Autodesk Inventor part; units mm, degrees
ref_plane "YZ Plane" through (0, 0, 0) normal (1, 0, 0) x (0, 1, 0)
ref_plane "XZ Plane" through (0, 0, 0) normal (0, 1, 0) x (-1, 0, 0)
ref_plane "XY Plane" through (0, 0, 0) normal (0, 0, 1) x (1, 0, 0)
sketch "Sketch1" plane through (0, 0, 0) normal (0, 1, 0) x (-1, 0, 0)
  circle A0 centre (0, 0) radius 10
  dimension "d0" = 20
extrude "Extrusion1" add sketch "Sketch1" along normal blind 15
sketch "Sketch2" plane through (0, 0, 0) normal (0, -1, 0) x (1, 0, 0)
  circle A0 centre (0, 0) radius 7.5
  dimension "d3" = 15
extrude "Extrusion2" cut sketch "Sketch2" against normal blind 5
fillet "Fillet1" radius 2 1 edges at (10, 15, 0)
sketch "Sketch3" plane through (0, 15, 0) normal (0, 1, 0) x (1, 0, 0)
  line L0 (-0.048, -4.9874) -> (-1.048, -4.9874)
  line L1 (-1.048, -4.9874) -> (-1.048, 2.5126)
  line L2 (-1.048, 2.5126) -> (-2.048, 2.5126)
  line L3 (-2.048, 2.5126) -> (-0.048, 5.0126)
  line L4 (-0.048, 5.0126) -> (-0.048, -4.9874)
  line L5 (-0.048, -4.9874) -> (0.952, -4.9874)
  line L6 (0.952, -4.9874) -> (0.952, 2.5126)
  line L7 (0.952, 2.5126) -> (1.952, 2.5126)
  line L8 (1.952, 2.5126) -> (-0.048, 5.0126)
  point P0 (0, 0)
  dimension "d7" = 1
  dimension "d8" = 7.5
  dimension "d9" = 10
extrude "Extrusion3" add sketch "Sketch3" along normal blind 0.5
properties part number "Device Direction Button"
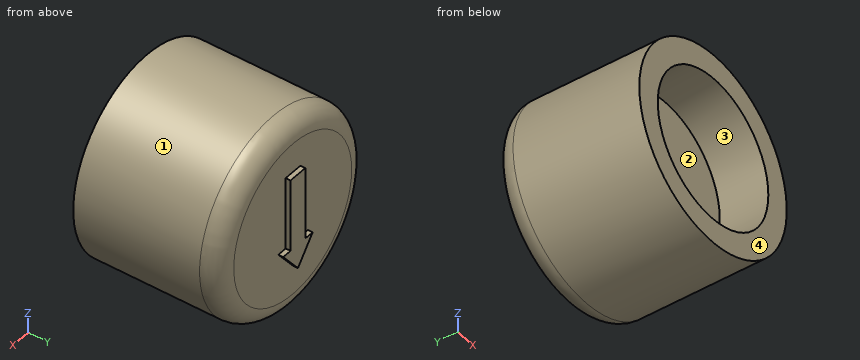
Input: part model. Units: mm. Frame: model coordinates. Face numbers are marked on the shaded views. Round coordinates to 2 decimals unless told otherwise and drop trailing zeros. Loops run counter-clockwise (first coordinate to the right, second up) from the corner with the lowest first, then second, coordinate; pieces in that order, holes last. Notation, with made-up numbers: M 18,31 L 22,31 A24 ccw 22,48 Z; hole C 69.5,-7 d3. An arc over 180 degrees is marked long. Answer in a Markdown table with one row per item. Add a question column.
1. Section A-A (z = 0). Output: boundary loops of the cut face in (x, y), and give its area (3 significant figures).
2. Section C-C (y = 11). Output: boundary loops of the cut face in (x, z), and give its area (3 significant figures).
3. Section B-B (y = 1). Output: boundary loops of the cut face in (x, z).
4. Mould query, pull axis Z, two halves, no side actions, for the marked faces 1, 2, 3 and 4. Classes: released by +Z, released by -Z, zero draft, split by the parting line, or undercut.
5. Contact query for flat-ended pins moving along their axis: pin 1 (3 mm diameter, centred on x = 0.5, z = -5.5, fed in from -Y); pin 2 (0.6 mm diameter, centred on y = 15, z = 2.5, fed in from +X); pin 3 (0.6 mm diameter, centred on y = 15.5, z = 3, fed in from -X). Output: stop coordinate, or through.
6. Ray query, probe 1 along Z at (x, y) = (0, 2.4); probe 2 along Y at (x, z) = (1.5, 5); probe 3 along Y at (x, z) = (0.75, -2.25). Return the intervals inside material, ascending.
Values follow:
| question | item | result |
|---|---|---|
| 1 | outline | M -10,0 L -7.5,0 L -7.5,5 L 7.5,5 L 7.5,0 L 10,0 L 10,13 A2 ccw 8,15 L 0.95,15 L 0.95,15.5 L -1.05,15.5 L -1.05,15 L -8,15 A2 ccw -10,13 Z |
| 1 | area | 224 mm^2 |
| 2 | outline | C 0,0 d20 |
| 2 | area | 314 mm^2 |
| 3 | outline | C 0,0 d20; hole C 0,0 d15 |
| 4 | face 1 | split by the parting line |
| 4 | face 2 | undercut |
| 4 | face 3 | undercut |
| 4 | face 4 | zero draft |
| 5 | pin 1 | y = 5 |
| 5 | pin 2 | x = 8.71 |
| 5 | pin 3 | x = -1.05 |
| 6 | probe 1 | -10 to -7.5, 7.5 to 10 |
| 6 | probe 2 | 5 to 15 |
| 6 | probe 3 | 5 to 15.5 |
